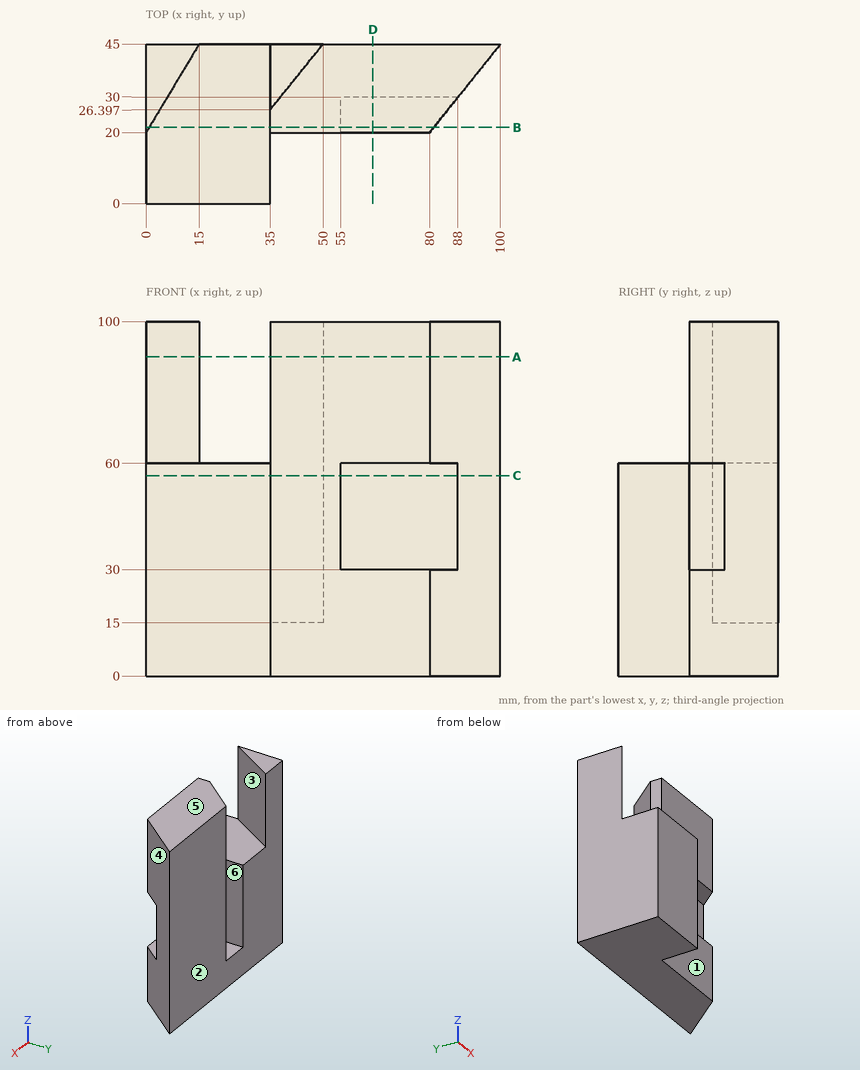
Can you work these out from the drawing? Everything is in mm from the part's minimum corner. A direction names the side the tool comes from. Give positions to 0.01 mm unless a question says otherwise; leave off trailing zeros. Loops run counter-clockwise (first coordinate to the right, second up) from the corner with the lowest first, then second, coordinate; pieces in that order, holes last. Notation, with made-up numbers: (36.5, -6) -> (95.5, -6) arc R21 cw to (95.5, 25) -> close; hole circle Ø6 at (80, 35.25). An arc over 180 degrees is marked (long way). Put each result on its own line as item: value.
(1) Imagine slicing it at C-C on z = 56.5. Write out the boundary of the cut face in (x, y), plus the area to 3 significant figures.
Computed:
outline: (0, 0) -> (35, 0) -> (35, 20) -> (55, 20) -> (55, 30) -> (88, 30) -> (100, 45) -> (50, 45) -> (35, 26.4) -> (35, 45) -> (0, 45) -> close
area: 2,520 mm^2
(2) Imagine slicing it at B-B on y = 21.5. Write out the boundary of the cut face in (x, z).
Computed:
outline: (0, 0) -> (81.2, 0) -> (81.2, 30) -> (55, 30) -> (55, 60) -> (81.2, 60) -> (81.2, 100) -> (35, 100) -> (35, 60) -> (0.9, 60) -> (0.9, 100) -> (0, 100) -> close
(3) Thinking about a two-plate mould opening in X: for the marked faces 4, 5 and 6, which applies, pulls with the +X half, pulls with the -X half, needs draft (parallel to the pull), parting line crosses it, or undercut?
Computed:
face 4: pulls with the +X half
face 5: needs draft
face 6: undercut
(4) Please list where these lines run through material, in increasing order: probe 1 along X at (y, z) = (29, 31); probe 2 along X at (y, z) = (14, 35.5); probe 3 along Z at (x, y) = (25.5, 19.5). Write a range as [from, to].
Computed:
probe 1: [0, 35], [37.1, 55]
probe 2: [0, 35]
probe 3: [0, 60]
(5) Imagine slicing it at D-D on x = 64. Write out the boundary of the cut face in (y, z), plus the area to 3 significant figures.
Computed:
outline: (20, 0) -> (45, 0) -> (45, 100) -> (20, 100) -> (20, 60) -> (30, 60) -> (30, 30) -> (20, 30) -> close
area: 2,200 mm^2
(6) For the marked faces 1, 2 and 3, which set-ups out of +Z, -Z, +X, -X, +Y, -Y let a thin tool reach every point of the face, with its end or its side?
Computed:
face 1: +Z, -Z, +X, -Y
face 2: +Z, -Z, +X, -X, +Y
face 3: +Z, -Y
(7) I'm going to push flat-ended pins straight in: pin 1 Ø3 at (y, z) = (22.5, 42) entering from +X; pin 2 Ø17.5 at (x, y) = (20, 15.5) entering from +Z; pin 3 Ø10 at (y, z) = (14.5, 44.5) entering from +X. Where does each tip first touch, or does it pass through?
Computed:
pin 1: x = 55
pin 2: z = 60
pin 3: x = 35
(8) Imagine slicing it at A-A on z = 90. Write out the boundary of the cut face in (x, y).
Computed:
outline: (0, 20) -> (15, 45) -> (0, 45) -> close; (35, 20) -> (80, 20) -> (100, 45) -> (50, 45) -> (35, 26.4) -> close
